Input: part model. Units: mm. Frame: model coordinates. Face numbers are marked on the shaded views. A direction names the side the tool comes from. Coordinates: 2 decimals unless noted, no trailing zeros. Write each loop counter-clockwise with the first axis right and the second up, starting at its lowest first coordinate (ties: lowest second). Pieces come first, ordered by that corner, then holes. Notation, with made-up numbers: M 10.5,14.5 L 38.5,14.5 A27 cw 38.5,35.5 Z; hole C -33,69.5 d8. An arc over 180 degrees is marked long. Write each question's results on one line, items separated by ' | '. Start each with the question number.
1. First-contact query: pin 1 (6 mm diameter, centred on x = -49, z = -7, fed in from +Y); pin 2 (3 mm diameter, centred on y = -11, z = 9.5, fed in from +X); pin 3 (6 mm diameter, centred on y = -5, z = -5, fed in from -X); pin 4 (7.5 mm diameter, centred on x = -53.5, y = -5.5, fed in from +Z). Flat tips, straight axial feed; report the tip coordinate or a pass-through.
2. Set-up query: the marked faces 1, 2 and 3. Return all of +Z, -Z, +X, -X, +Y, -Y with unobstructed straight access to the full face (end or side cutting, diameter ignored); none if empty.
3. Ray query, probe 1 along Z at (x, y) = (-39.5, -2.25); probe 2 along X at (y, z) = (-13, 0); probe 3 along Z at (x, y) = (25.5, -8.5). Return the intervals inside material, ascending.
4. Section query B-B, the plane y = -6.25. Count the separate pieces of the cut face and the enclosed holes in it, and give its area (3 significant figures).
5. Pull-direction query (X, two-part tool) for the marked faces 4, 5, 6 and 7; classes: +X half, -X half, draft (parallel to the pull), parting line (faces both ways), or undercut.
6. Section query A-A, the plane x = 10. Output: boundary loops of the cut face in (y, z).
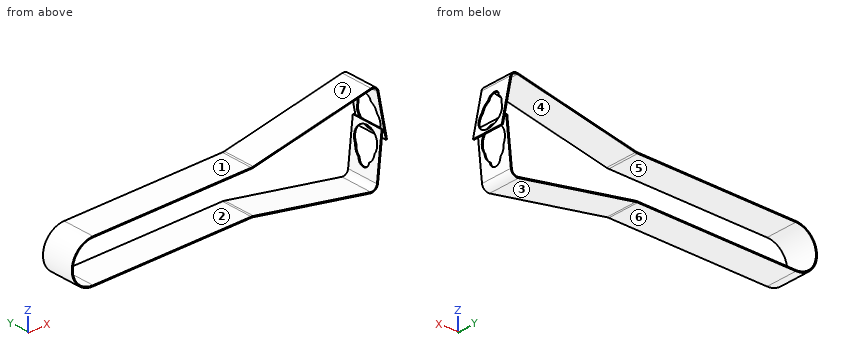
```python
from build123d import *

# Parameters (mm, degrees)
F1_DEPTH = 15
F3_DEPTH = 0.5
F5_DEPTH = 1


with BuildPart() as f1:
    # F0 (on Front) → F1 (new body)
    with BuildSketch(Plane.XZ):
        with BuildLine():
            Line((-0.481445241, 10), (-75, 10))
            ThreePointArc((-75, 10), (-85, 0), (-75, -10))
            Line((-75, -10), (-0.481445241, -10))
            ThreePointArc((-0.481445241, -10), (-0.0022164784, -10.0230190082), (0.4725997359, -10.0918640828))
            Line((0.4725997359, -10.0918640828), (55.6838567363, -20.8238452864))
            ThreePointArc((55.6838567363, -20.8238452864), (58.0407520827, -20.2905343179), (59.2398494086, -18.1925491258))
            Line((59.2398494086, -18.1925491258), (61.4349471372, 2.6924106769))
            Line((61.4349471372, 2.6924106769), (60.9376861895, 2.7446749085))
            Line((60.9376861895, 2.7446749085), (58.7425884609, -18.1402848942))
            ThreePointArc((58.7425884609, -18.1402848942), (57.7433406893, -19.8886058876), (55.779261234, -20.3330316947))
            Line((55.779261234, -20.3330316947), (0.5680042336, -9.601050491))
            ThreePointArc((0.5680042336, -9.601050491), (0.0457063979, -9.525320909), (-0.481445241, -9.5))
            Line((-0.481445241, -9.5), (-75, -9.5))
            ThreePointArc((-75, -9.5), (-84.5, 0), (-75, 9.5))
            Line((-75, 9.5), (-0.481445241, 9.5))
            ThreePointArc((-0.481445241, 9.5), (0.0457063979, 9.525320909), (0.5680042336, 9.601050491))
            Line((0.5680042336, 9.601050491), (56.0481539542, 20.3852991447))
            ThreePointArc((56.0481539542, 20.3852991447), (57.9231587013, 20.0038251175), (58.9792444013, 18.4082536746))
            Line((58.9792444013, 18.4082536746), (62.9862333042, -2.2059171778))
            Line((62.9862333042, -2.2059171778), (63.4770468959, -2.1105126802))
            Line((63.4770468959, -2.1105126802), (59.470057993, 18.5036581722))
            ThreePointArc((59.470057993, 18.5036581722), (58.2027551531, 20.4183439038), (55.9527494565, 20.8761127365))
            Line((55.9527494565, 20.8761127365), (0.4725997359, 10.0918640828))
            ThreePointArc((0.4725997359, 10.0918640828), (-0.0022164784, 10.0230190082), (-0.481445241, 10))
        make_face()
    extrude(amount=F1_DEPTH)

    # F2 (on face) → F3 (cut)
    with BuildSketch(Plane(origin=(60.7706639739, 0, 11.8126204498), x_dir=(0, 1, 0), z_dir=(0.9816271834, 0, 0.1908089954))):
        with BuildLine():
            ThreePointArc((-4.75, 0.4920951066), (-7.5, 3.2420951066), (-10.25, 0.4920951066))
            ThreePointArc((-10.25, 0.4920951066), (-11.9017042154, -1.3120199204), (-12.5, -3.6837281655))
            ThreePointArc((-12.5, -3.6837281655), (-7.5, -13.0003529559), (-2.5, -3.6837281655))
            ThreePointArc((-2.5, -3.6837281655), (-3.0982957846, -1.3120199204), (-4.75, 0.4920951066))
        make_face()
    extrude(amount=-F3_DEPTH, mode=Mode.SUBTRACT)

    # F4 (on face) → F5 (cut)
    with BuildSketch(Plane(origin=(60.4838048122, 0, -6.3571040507), x_dir=(0, 1, 0), z_dir=(0.9945218954, 0, -0.1045284633))):
        with BuildLine():
            ThreePointArc((-2.5, -1.4006380153), (-7.5, 7.915986775), (-12.5, -1.4006380153))
            ThreePointArc((-12.5, -1.4006380153), (-11.9017042154, -3.7723462605), (-10.25, -5.5764612875))
            ThreePointArc((-10.25, -5.5764612875), (-7.5, -8.3264612875), (-4.75, -5.5764612875))
            ThreePointArc((-4.75, -5.5764612875), (-3.0982957846, -3.7723462605), (-2.5, -1.4006380153))
        make_face()
    extrude(amount=-F5_DEPTH, mode=Mode.SUBTRACT)


solid = f1.part
```
Answer:
1) pin 1: y = 0 | pin 2: x = 61.31 | pin 3: x = -84.8 | pin 4: z = 10
2) face 1: +Z, -X, +Y, -Y | face 2: +Y, -Y | face 3: -Z, -X, +Y, -Y
3) probe 1: -10 to -9.5, 9.5 to 10 | probe 2: -85 to -84.5, 60.65 to 61.15, 62.56 to 63.07 | probe 3: -14.96 to -14.45, 14.45 to 14.96
4) separate pieces: 3 | enclosed holes: 0 | area: 157 mm^2
5) face 4: undercut | face 5: undercut | face 6: draft | face 7: -X half
6) outline: M -15,-11.94 L 0,-11.94 L 0,-11.43 L -15,-11.43 Z; M -15,11.43 L 0,11.43 L 0,11.94 L -15,11.94 Z
